Geometry check sheet. Reference: the model listing, model coordinates, mm. A direction names the side the tool comes from. Round coordinates to 2 decimals unless told otherwise and drop trailing zeros. Put each result on its own line as item: value. Start each with the question number.
(1) Tool access check on faces 4 (the flat face through (-1, 1, -34.705)), 5 (the flat face through (27.085, 1, 1)), 6 (the flat face through (60.952, 1, 1)). Record the directions out of +Z, -Z, +X, -X, +Y, -Y that give a thin tool (end or side, any length) a straight path to the whole face; none if there is none.
(2) Section check A-A on y = 1.6. Count the separate pieces of the cut face and the enclosed holes in it, then the cut area to 3 significant figures.
(3) Material ranges on probe 1 along X at (y, z) = (0.45, -3); probe 2 along Z at (x, y) = (42, 2.8); probe 3 along X at (y, z) = (0.3, -25.5), recorded low to high.
(4) Mould release check, pull along X, two halves, no side actions. Record for faces 1 (the flat face through (-2, 1, -60.952)), 2 (the flat face through (34.705, 1, 2)), 3 (the flat face through (0, 1, -48)): pulls with the +X half, pulls with the -X half, needs draft (parallel to the pull), parting line crosses it, or undercut.
(5) Gauge pin test, flat ends, axial feed: pin 1 (0.9 mm diameter, centred on y = 2, z = -53.5, fed in from -X); pin 2 (3.5 mm diameter, centred on x = -0.25, z = -64.76, fed in from +Y); pin 3 (1 mm diameter, centred on x = 23.5, y = 0.5, fed in from -Z); pin 4 (1.5 mm diameter, centred on x = 8, y = 1, fed in from +Z). Record the tip position at first contact, or that the pin passes through.
from build123d import *

# Parameters (mm, degrees)
EXTRUDE_1_DEPTH = 2.9718


with BuildPart() as part:
    # 草图1 → 凸台-拉伸1 (new body)
    with BuildSketch(Plane(origin=(0, 0, 0), x_dir=(1, 0, 0), z_dir=(0, 1, 0))):
        with BuildLine():
            Line((0, 60.951533333), (0, 34.704866667))
            Line((0, 34.704866667), (0, 32.878672101))
            ThreePointArc((0, 32.878672101), (1.247332741, 32.216229599), (1.746, 30.894866667))
            ThreePointArc((1.746, 30.894866667), (1.247332741, 29.573503734), (0, 28.911061233))
            Line((0, 28.911061233), (0, 27.084866667))
            Line((0, 27.084866667), (0, 0))
            Line((0, 0), (27.084866667, 0))
            Line((27.084866667, 0), (28.911061233, 0))
            ThreePointArc((28.911061233, 0), (30.894866667, 1.746), (32.878672101, 0))
            Line((32.878672101, 0), (34.704866667, 0))
            Line((34.704866667, 0), (60.951533333, 0))
            Line((60.951533333, 0), (62.777727899, 0))
            ThreePointArc((62.777727899, 0), (64.761533333, 1.746), (66.745338767, 0))
            Line((66.745338767, 0), (68.571533333, 0))
            Line((68.571533333, 0), (98.6282, 0))
            Line((98.6282, 0), (98.6282, 5.08))
            add(Edge.make_bspline(
                [(5.08, 98.6282), (49.328709516, 96.847818465), (96.847818465, 49.328709516), (98.6282, 5.08)],
                knots=[0.03565985, 0.03565985, 0.03565985, 0.03565985, 0.96434015, 0.96434015, 0.96434015, 0.96434015], degree=3))
            Line((5.08, 98.6282), (0, 98.6282))
            Line((0, 98.6282), (0, 68.571533333))
            Line((0, 68.571533333), (0, 66.745338767))
            ThreePointArc((0, 66.745338767), (1.247332741, 66.082896266), (1.746, 64.761533333))
            ThreePointArc((1.746, 64.761533333), (1.247332741, 63.440170401), (0, 62.777727899))
            Line((0, 62.777727899), (0, 60.951533333))
        make_face()
        with BuildLine():
            Line((-2.9718, 60.951533333), (0, 60.951533333))
            Line((0, 60.951533333), (0, 62.777727899))
            ThreePointArc((0, 62.777727899), (-2.254, 64.761533333), (0, 66.745338767))
            Line((0, 66.745338767), (0, 68.571533333))
            Line((0, 68.571533333), (-2.9718, 68.571533333))
            Line((-2.9718, 68.571533333), (-2.9718, 60.951533333))
        make_face()
        with BuildLine():
            Line((0, 32.878672101), (0, 34.704866667))
            Line((0, 34.704866667), (-2.9718, 34.704866667))
            Line((-2.9718, 34.704866667), (-2.9718, 27.084866667))
            Line((-2.9718, 27.084866667), (0, 27.084866667))
            Line((0, 27.084866667), (0, 28.911061233))
            ThreePointArc((0, 28.911061233), (-2.254, 30.894866667), (0, 32.878672101))
        make_face()
        with BuildLine():
            Line((28.911061233, 0), (27.084866667, 0))
            Line((27.084866667, 0), (27.084866667, -2.9718))
            Line((27.084866667, -2.9718), (34.704866667, -2.9718))
            Line((34.704866667, -2.9718), (34.704866667, 0))
            Line((34.704866667, 0), (32.878672101, 0))
            ThreePointArc((32.878672101, 0), (32.890813919, -0.126742128), (32.894866667, -0.254))
            ThreePointArc((32.894866667, -0.254), (30.767608795, -2.249947252), (28.911061233, 0))
        make_face()
        with BuildLine():
            Line((62.777727899, 0), (60.951533333, 0))
            Line((60.951533333, 0), (60.951533333, -2.9718))
            Line((60.951533333, -2.9718), (68.571533333, -2.9718))
            Line((68.571533333, -2.9718), (68.571533333, 0))
            Line((68.571533333, 0), (66.745338767, 0))
            ThreePointArc((66.745338767, 0), (66.757480586, -0.126742128), (66.761533333, -0.254))
            ThreePointArc((66.761533333, -0.254), (64.634275461, -2.249947252), (62.777727899, 0))
        make_face()
    extrude(amount=EXTRUDE_1_DEPTH)


solid = part.part
Answers follow:
1. face 4: -X, +Y, -Y
1. face 5: +Z, -X, +Y, -Y
1. face 6: +Z, +Y, -Y
2. separate pieces: 1
2. enclosed holes: 4
2. area: 7,480 mm^2
3. probe 1: x = 0 to 98.63
3. probe 2: z = -87.42 to 0
3. probe 3: x = 0 to 94.76
4. face 1: needs draft
4. face 2: undercut
4. face 3: pulls with the -X half
5. pin 1: stops at x = 0
5. pin 2: passes through
5. pin 3: stops at z = -95.54
5. pin 4: stops at z = 0
